Verification items for the finished model (mm, model axes). A direction names the side the tool comes from. Coordinates: 2 decimals unless noted, no trailing zeros. Write each loop counter-clockwise with the first axis right and the second up, starting at its lowest first coordinate (ties: lowest second). Pieces come first, ordered by that corner, then holes. Notation, with made-up numbers: (-15.5, -33.5) - (15.5, -33.5) arc R18 cw to (15.5, -27.5) - close; hole circle Ø4 at (7.25, 89). An arc over 180 degrees is marked (long way). Use CSV: the item, a comma, the result in double quotes. Start each with the question number.
```python
from build123d import *

# Parameters (mm, degrees)
CROQUIS1_W                    = 100
CROQUIS1_H                    = 173
CROQUIS1_R                    = 1.5
SALIENTE_EXTRUIR7_DEPTH       = 3
CROQUIS1_13_W                 = 100
CROQUIS1_13_H                 = 173
SALIENTE_EXTRUIR8_DEPTH       = 5
CROQUIS1_16_W                 = 106
CROQUIS1_16_H                 = 179
CROQUIS1_16_W_2               = 100
CROQUIS1_16_H_2               = 173
SALIENTE_EXTRUIR9_DEPTH       = 90
REDONDEO1_R                   = 3
CROQUIS4_W                    = 37
CROQUIS4_H                    = 150
CROQUIS4_R                    = 7.5
CROQUIS4_R_2                  = 8.5
SALIENTE_EXTRUIR10_DEPTH      = 5
SALIENTE_EXTRUIR11_DEPTH      = 50
SALIENTE_EXTRUIR11_DEPTH_BACK = 50
REDONDEO2_R                   = 10
CROQUIS1_17_R                 = 1.5
CROQUIS1_17_W                 = 7
CROQUIS1_17_H                 = 100
SALIENTE_EXTRUIR12_DEPTH      = 55
CROQUIS12_W                   = 60
CROQUIS12_H                   = 3
SALIENTE_EXTRUIR13_DEPTH      = 7
CROQUIS16_R                   = 1.5
CORTAR_EXTRUIR5_DEPTH         = 10
CROQUIS17_R                   = 2
CORTAR_EXTRUIR6_DEPTH         = 10
CROQUIS19_R                   = 3.5
CROQUIS19_R_2                 = 5
CORTAR_EXTRUIR7_DEPTH         = 10
REDONDEO3_R                   = 60
REDONDEO4_START               = -30
REDONDEO4_DEPTH               = 28.499998795
REDONDEO4_START_2             = 1.500002077
REDONDEO4_2_DEPTH             = 28.499997923
REDONDEO4_START_3             = -1.500001205
REDONDEO4_3_DEPTH             = 3.000003282
REDONDEO4_START_4             = 23.875277779
REDONDEO4_4_OUTLINE_R         = 1.5
REDONDEO4_4_DEPTH             = 28.124722221


with BuildPart() as part:
    # Croquis1 → Saliente-Extruir7 (new body)
    with BuildSketch(Plane(origin=(0, 0, 0), x_dir=(1, 0, 0), z_dir=(0, 1, 0))):
        Rectangle(CROQUIS1_W, CROQUIS1_H)
        with Locations(Location((-36, -23.5, 0), (0, 0, 270))):
            Circle(CROQUIS1_R, mode=Mode.SUBTRACT)
        with Locations(Location((36, -23.5, 0), (0, 0, 270))):
            Circle(CROQUIS1_R, mode=Mode.SUBTRACT)
    extrude(amount=SALIENTE_EXTRUIR7_DEPTH)

    # Croquis1<13> → Saliente-Extruir8 (add)
    with BuildSketch(Plane(origin=(0, 0, 0), x_dir=(1, 0, 0), z_dir=(0, 1, 0))):
        Rectangle(CROQUIS1_13_W, CROQUIS1_13_H)
    extrude(amount=SALIENTE_EXTRUIR8_DEPTH)

    # Croquis1<16> → Saliente-Extruir9 (add)
    with BuildSketch(Plane(origin=(0, 0, 0), x_dir=(1, 0, 0), z_dir=(0, 1, 0))):
        Rectangle(CROQUIS1_16_W, CROQUIS1_16_H)
        Rectangle(CROQUIS1_16_W_2, CROQUIS1_16_H_2, mode=Mode.SUBTRACT)
    extrude(amount=SALIENTE_EXTRUIR9_DEPTH)

    # Redondeo1
    redondeo1_edges = [part.edges().sort_by_distance(p)[0] for p in [
        (-53, 45, 89.5),
        (53, 45, 89.5),
        (53, 45, -89.5),
        (-53, 45, -89.5),
    ]]
    fillet(redondeo1_edges, radius=REDONDEO1_R)

    # Croquis4 → Saliente-Extruir10 (add)
    # profile 1 of 2: a face of its own
    with BuildSketch(Plane(origin=(0, 0, 0), x_dir=(1, 0, 0), z_dir=(0, 1, 0))):
        with Locations((-71.5, 0)):
            Rectangle(CROQUIS4_W, CROQUIS4_H)
    # profile 2 of 2: a face of its own
    with BuildSketch(Plane(origin=(0, 0, 0), x_dir=(1, 0, 0), z_dir=(0, 1, 0))):
        with Locations((71.5, 0)):
            Rectangle(CROQUIS4_W, CROQUIS4_H)
        with Locations(Location((73, 25, 0), (0, 0, 270))):
            Circle(CROQUIS4_R, mode=Mode.SUBTRACT)
        with Locations(Location((73, -25, 0), (0, 0, 270))):
            Circle(CROQUIS4_R_2, mode=Mode.SUBTRACT)
    extrude(amount=SALIENTE_EXTRUIR10_DEPTH)

    # Croquis5 → Saliente-Extruir11 (add, two sides: drawn at the far end of the back side and taken through both)
    with BuildSketch(Plane.XY.offset(-SALIENTE_EXTRUIR11_DEPTH_BACK)):
        Polygon((-53, 5), (-53, 20), (-63, 5), align=None)
        Polygon((53, 5), (53, 20), (63, 5), align=None)
    extrude(amount=SALIENTE_EXTRUIR11_DEPTH + SALIENTE_EXTRUIR11_DEPTH_BACK)

    # Redondeo2
    redondeo2_edges = [part.edges().sort_by_distance(p)[0] for p in [
        (90, 2.5, 75),
        (90, 2.5, -75),
        (-90, 2.5, -75),
        (-90, 2.5, 75),
    ]]
    fillet(redondeo2_edges, radius=REDONDEO2_R)

    # Croquis1<17> → Saliente-Extruir12 (add)
    # profile 1 of 2: a face of its own
    with BuildSketch(Plane(origin=(0, 0, 0), x_dir=(1, 0, 0), z_dir=(0, 1, 0))):
        Polygon((32.5, -73.5), (0, -73.5), (0, -75.5), (39.5, -75.5), (39.5, 26.5), (32.5, 26.5), align=None)
        with Locations(Location((36, -23.5, 0), (0, 0, 90))):
            Circle(CROQUIS1_17_R, mode=Mode.SUBTRACT)
    # profile 2 of 2: a face of its own
    with BuildSketch(Plane(origin=(0, 0, 0), x_dir=(1, 0, 0), z_dir=(0, 1, 0))):
        with Locations((-36, -23.5)):
            Rectangle(CROQUIS1_17_W, CROQUIS1_17_H)
        with Locations(Location((-36, -23.5, 0), (0, 0, 90))):
            Circle(CROQUIS1_17_R, mode=Mode.SUBTRACT)
    extrude(amount=SALIENTE_EXTRUIR12_DEPTH)

    # Croquis12 → Saliente-Extruir13 (add)
    with BuildSketch(Plane.XY.offset(-86.5)):
        with Locations((0, 53.5)):
            Rectangle(CROQUIS12_W, CROQUIS12_H)
    extrude(amount=SALIENTE_EXTRUIR13_DEPTH)

    # Croquis16 → Cortar-Extruir5 (cut)
    with BuildSketch(Plane(origin=(0, 55, 0), x_dir=(1, 0, 0), z_dir=(0, 1, 0))):
        with Locations(Location((0, 83, 0), (0, 0, 180))):
            Circle(CROQUIS16_R)
    extrude(amount=-CORTAR_EXTRUIR5_DEPTH, mode=Mode.SUBTRACT)

    # Croquis17 → Cortar-Extruir6 (cut)
    with BuildSketch(Plane(origin=(0, 5, 0), x_dir=(1, 0, 0), z_dir=(0, 1, 0))):
        with Locations(Location((-65.5, 62.5, 0), (0, 0, 270))):
            Circle(CROQUIS17_R)
        with Locations(Location((65.5, 62.5, 0), (0, 0, 270))):
            Circle(CROQUIS17_R)
        with Locations(Location((65.5, -62.5, 0), (0, 0, 270))):
            Circle(CROQUIS17_R)
        with Locations(Location((-65.5, -62.5, 0), (0, 0, 270))):
            Circle(CROQUIS17_R)
    extrude(amount=-CORTAR_EXTRUIR6_DEPTH, mode=Mode.SUBTRACT)

    # Croquis19 → Cortar-Extruir7 (cut)
    with BuildSketch(Plane(origin=(0, 5, 0), x_dir=(1, 0, 0), z_dir=(0, 1, 0))):
        with Locations(Location((-73, 25, 0), (0, 0, 270))):
            Circle(CROQUIS19_R)
        with Locations(Location((-71.5, -25, 0), (0, 0, 270))):
            Circle(CROQUIS19_R_2)
    extrude(amount=-CORTAR_EXTRUIR7_DEPTH, mode=Mode.SUBTRACT)

    # Redondeo3
    # the kernel refuses this fillet: 60 mm, written as the material it adds along each edge
    with BuildSketch(Plane(origin=(53, 20, 50), x_dir=(0, 1, 0), z_dir=(0, 0, -1)), Plane(origin=(-53, 20, -50), x_dir=(0, 1, 0), z_dir=(0, 0, 1))) as redondeo3_piece_1:
        with BuildLine():
            CenterArc((REDONDEO3_R * 0.302775637732, REDONDEO3_R), REDONDEO3_R, 236.309932474, 33.690067526)
            Line((-REDONDEO3_R * 0.251924558493, REDONDEO3_R * 0.167949705662), (0, 0))
            Line((0, 0), (REDONDEO3_R * 0.302775637732, 0))
        make_face()
    extrude(amount=100)

    # Redondeo4: read off the stored shape, not the designer's step
    # Redondeo4 outline → Redondeo4 (add)
    with BuildSketch(Plane.YZ.offset(REDONDEO4_START)):
        with BuildLine():
            ThreePointArc((52, -79.5), (38.366654525, -84.723706512), (23.875277779, -86.5))
            Line((23.875277779, -86.5), (52, -86.5))
            Line((52, -86.5), (52, -79.5))
        make_face()
    extrude(amount=REDONDEO4_DEPTH)

    # Redondeo4 2 outline → Redondeo4 2 (add)
    with BuildSketch(Plane.YZ.offset(REDONDEO4_START_2)):
        with BuildLine():
            ThreePointArc((52, -79.5), (38.366654525, -84.723706512), (23.875277779, -86.5))
            Line((23.875277779, -86.5), (52, -86.5))
            Line((52, -86.5), (52, -79.5))
        make_face()
    extrude(amount=REDONDEO4_2_DEPTH)

    # Redondeo4 3 outline → Redondeo4 3 (add)
    with BuildSketch(Plane.YZ.offset(REDONDEO4_START_3)):
        with BuildLine():
            ThreePointArc((52, -79.5), (38.366654525, -84.723706512), (23.875277779, -86.5))
            Line((23.875277779, -86.5), (52, -86.5))
            Line((52, -86.5), (52, -79.5))
        make_face()
    extrude(amount=REDONDEO4_3_DEPTH)

    # Redondeo4 4 outline → Redondeo4 4 (cut)
    with BuildSketch(Plane(origin=(0, 0, 0), x_dir=(1, 0, 0), z_dir=(0, 1, 0)).offset(REDONDEO4_START_4)):
        with Locations((0, 83)):
            Circle(REDONDEO4_4_OUTLINE_R)
    extrude(amount=REDONDEO4_4_DEPTH, mode=Mode.SUBTRACT)


solid = part.part
```
Q1. Cross-section at A-A (y = 8.5). State how many separate pieces and enclosed holes the cut face has, plus the area to 3 significant figures.
Q2. Cross-section at D-D (x = -58). Record the cut outline in (y, z), plus the area to 3 significant figures.
Q3. Tool access check on faces 4 (the cylindrical face through (86.99, 2.54, 72.15)), 5 (the flat face through (-67, 2, -75)), 6 (the flat face through (50, 47, 1)). Record the directions out of +Z, -Z, +X, -X, +Y, -Y that give a thin tool (end or side, any length) a straight path to the whole face; none if there is none.
Q4. Cross-section at B-B (y = 78.5). Record the cut outline in (x, z).
Q5. Scan lines: line 1 along X through (y, z) = (47, 4); line 2 along X through (y, z) = (1, -25); line 3 along Z through (x, y) = (-36, 42). Record each from-to range of solid material in increasing order. Write a range as from..to.
Q6. Gauge pin test, flat ends, axial feed: pin 1 (3.5 mm diameter, centred on x = 35.5, z = 23, fed in from +Y); pin 2 (4 mm diameter, centred on x = -26, z = 66.5, fed in from +Y); pin 3 (18.5 mm diameter, centred on x = -72, z = 9.5, fed in from +Y); pin 4 (12 mm diameter, centred on x = 73, z = -25, fed in from -Y). Record the tip position at first contact, or that the pin passes through.
Q7. Release check for a two-part mould opening along Y. For faces 1 (the flat face through (-1, 56, -86.5)), 2 (the flat face through (-34, 55, 23)), 3 (the flat face through (-56, 12, 50)) record: released by +Y, released by -Y, zero draft, split by the parting line, or undercut.
Q8. Cross-section at C-C (z = -3). Record the cut outline in (x, y).
Reply:
1,separate pieces,"3"
1,enclosed holes,"3"
1,area,"4,700 mm^2"
2,outline,"(0, -75) - (5, -75) - (5, -50) - (14.19, -50) - (14.19, 50) - (5, 50) - (5, 75) - (0, 75) - close"
2,area,"1,670 mm^2"
3,face 4,"+Z, +X, +Y, -Y"
3,face 5,"-Z, -X, +Y, -Y"
3,face 6,"+Y"
4,outline,"(-53, -86.5) arc R3 ccw to (-50, -89.5) - (50, -89.5) arc R3 ccw to (53, -86.5) - (53, 86.5) arc R3 ccw to (50, 89.5) - (-50, 89.5) arc R3 ccw to (-53, 86.5) - close; hole (-50, -86.5) - (50, -86.5) - (50, 86.5) - (-50, 86.5) - close"
5,line 1,"-53..-50, -39.5..-32.5, 32.5..39.5, 50..53"
5,line 2,"-90..-76.5, -69.5..65.5, 80.5..90"
5,line 3,"-89.5..-86.5, -26.5..22, 25..73.5, 86.5..89.5"
6,pin 1,"y = 55"
6,pin 2,"y = 5"
6,pin 3,"y = 5.38"
6,pin 4,"through"
7,face 1,"undercut"
7,face 2,"released by +Y"
7,face 3,"zero draft"
8,outline,"(-90, 0) - (90, 0) - (90, 5) - (63, 5) arc R60 cw to (53, 38.17) - (53, 90) - (50, 90) - (50, 5) - (39.5, 5) - (39.5, 55) - (32.5, 55) - (32.5, 5) - (-32.5, 5) - (-32.5, 55) - (-39.5, 55) - (-39.5, 5) - (-50, 5) - (-50, 90) - (-53, 90) - (-53, 38.17) arc R60 cw to (-63, 5) - (-90, 5) - close"
